The listing builds one solid part. Answer for the finished solid, in the listing's coordinates (mm). A direction names the side the tool comes from. Round coordinates to 2 decimals unless told otherwise and drop trailing zeros. Write each loop counter-clockwise with the first axis right and the second up, starting at its lowest first coordinate (ties: lowest second). Pieces come first, ordered by that corner, then holes. Notation, with made-up numbers: (-31, 14) - (21, 14) arc R23 ccw to (21, 45) - close; hole circle Ø4 at (37, -33). An arc over 180 degrees is marked (long way). Return JSON: item names as keys, results as strings. Group by question number.
from build123d import *

# Parameters (mm, degrees)
SKETCH_1_W          = 60
SKETCH_1_H          = 50
SKETCH_1_W_2        = 29.5
SKETCH_1_H_2        = 22.5
EXTRUDE_1_DEPTH     = 2.5
SKETCH_8_R          = 1.55
CUT_EXTRUDE_2_DEPTH = 10
FILLET_1_R          = 1
FILLET_2_R          = 12


with BuildPart() as part:
    # 草图1 → 凸台-拉伸1 (new body)
    with BuildSketch(Plane(origin=(0, 0, 0), x_dir=(1, 0, 0), z_dir=(0, 1, 0))):
        Rectangle(SKETCH_1_W, SKETCH_1_H)
        Rectangle(SKETCH_1_W_2, SKETCH_1_H_2, mode=Mode.SUBTRACT)
    extrude(amount=EXTRUDE_1_DEPTH)

    # 草图8 → 切除-拉伸2 (cut)
    with BuildSketch(Plane.XZ):
        with Locations((27, 8)):
            Circle(SKETCH_8_R)
        with Locations((10, 22)):
            Circle(SKETCH_8_R)
        with Locations((-10, 22)):
            Circle(SKETCH_8_R)
        with Locations((-27, 8)):
            Circle(SKETCH_8_R)
        with Locations((-27, -8)):
            Circle(SKETCH_8_R)
        with Locations((-10, -22)):
            Circle(SKETCH_8_R)
        with Locations((10, -22)):
            Circle(SKETCH_8_R)
        with Locations((27, -8)):
            Circle(SKETCH_8_R)
    extrude(amount=-CUT_EXTRUDE_2_DEPTH, mode=Mode.SUBTRACT)

    # 圆角1
    fillet_1_edges = [part.edges().sort_by_distance(p)[0] for p in [
        (14.75, 1.25, 11.25),
        (14.75, 1.25, -11.25),
        (-14.75, 1.25, -11.25),
        (-14.75, 1.25, 11.25),
    ]]
    fillet(fillet_1_edges, radius=FILLET_1_R)

    # 圆角2
    fillet_2_edges = [part.edges().sort_by_distance(p)[0] for p in [
        (30, 1.25, 25),
        (-30, 1.25, 25),
        (-30, 1.25, -25),
        (30, 1.25, -25),
    ]]
    fillet(fillet_2_edges, radius=FILLET_2_R)


solid = part.part
(1) A flat-ended cylindrical pin translates along its axis: pin 1 (1.9 mm diameter, centred on x = -10, z = 22, fed in from +Y). Find the tip coordinate at first contact, or state that the pin passes through.
(2) Find section D-D (z = -1). Write down the section's boundary in (x, y), plus the area to 4 significant figures.
(3) Consider line 1 (Z direction, x = 10, y = 0.45); line 2 (X direction, y = 0.35, z = 6); line 3 (Z direction, x = 0.5, y = 1.9). Determine where each line is inside the solid, lowest interval first.
(4) Determine the mould class of faces 1 (the cylindrical face through (-25.568, 1.232, -8.594)), 2 (the flat face through (30, 1, 0)), 3 (the cylindrical face through (26.39, 1.27, 21.58)), 4 (the cylindrical face through (-10.202, 1.232, -20.463)) for opening direction Z: +Z half, -Z half, draft (parallel to the pull), parting line (faces both ways), or undercut.
(5) Find section B-B (y = 1.4). State how many separate pieces and enclosed holes the cut face has, plus the area to 3 significant figures.
(6) Find section C-C (x = 10). Write down the section's boundary in (y, z), plus the area to 4 significant figures.
(7) Find section A-A (z = -8). Write down the section's boundary in (x, y), plus the area to 4 significant figures.
(8) For faces 5 (the flat face through (0, 1, -11.25)), 6 (the cylindrical face through (-26.58, 1.27, 21.39)), determine the directions among +Z, -Z, +X, -X, +Y, -Y from which every point of the face is accessible in a straight line to the end or side of a thin tool.
Check sheet entries:
{
 "1": {"pin 1": "passes through"},
 "2": {"outline": "(-30, 0) - (-14.75, 0) - (-14.75, 2.5) - (-30, 2.5) - close; (14.75, 0) - (30, 0) - (30, 2.5) - (14.75, 2.5) - close", "area": "76.25 mm^2"},
 "3": {"line 1": "z = -25 to -23.55, -20.45 to -11.25, 11.25 to 20.45, 23.55 to 25", "line 2": "x = -30 to -14.75, 14.75 to 30", "line 3": "z = -25 to -11.25, 11.25 to 25"},
 "4": {"face 1": "undercut", "face 2": "draft", "face 3": "+Z half", "face 4": "undercut"},
 "5": {"separate pieces": "1", "enclosed holes": "9", "area": "2,150 mm^2"},
 "6": {"outline": "(0, -25) - (2.5, -25) - (2.5, -23.55) - (0, -23.55) - close; (0, -20.45) - (2.5, -20.45) - (2.5, -11.25) - (0, -11.25) - close; (0, 11.25) - (2.5, 11.25) - (2.5, 20.45) - (0, 20.45) - close; (0, 23.55) - (2.5, 23.55) - (2.5, 25) - (0, 25) - close", "area": "53.25 mm^2"},
 "7": {"outline": "(-30, 0) - (-28.55, 0) - (-28.55, 2.5) - (-30, 2.5) - close; (-25.45, 0) - (-14.75, 0) - (-14.75, 2.5) - (-25.45, 2.5) - close; (14.75, 0) - (25.45, 0) - (25.45, 2.5) - (14.75, 2.5) - close; (28.55, 0) - (30, 0) - (30, 2.5) - (28.55, 2.5) - close", "area": "60.75 mm^2"},
 "8": {"face 5": "+Y, -Y", "face 6": "+Z, -X, +Y, -Y"}
}
